Verification items for the finished model (mm, model axes). A direction names the side the tool comes from. Give positions to 0.01 mm unless a question says otherwise; leave off trailing zeros. Write each loop counter-clockwise with the first axis right and the second up, starting at its lowest first coordinate (ties: lowest second). Pieces come first, ordered by that corner, then holes.
Autodesk Inventor part; units mm, degrees
ref_plane "YZ Plane" through (0, 0, 0) normal (1, 0, 0) x (0, 1, 0)
ref_plane "XZ Plane" through (0, 0, 0) normal (0, 1, 0) x (-1, 0, 0)
ref_plane "XY Plane" through (0, 0, 0) normal (0, 0, 1) x (1, 0, 0)
sketch "Sketch1" plane through (0, 0, 0) normal (0, 1, 0) x (-1, 0, 0)
  line L0 (0, 18.5) -> (0, -18.5)
  line L1 (-4, 14.5) -> (-4, -14.5)
  line L2 (0, 0) -> (-19.6483, 0) construction
  line L3 (-4, 14.5) -> (0, 18.5)
  line L4 (0, -18.5) -> (-4, -14.5)
  point P0 (-4, 0)
  dimension "d6" = 37
  dimension "d7" = 29
  dimension "d8" = 4
extrude "Extrusion1" add sketch "Sketch1" along normal blind 18
sketch "Sketch2" plane through (4, 0, 14.5) normal (1, 0, 0) x (0, 0, -1)
  line L0 (-4, 0) -> (-4, 18)
  line L1 (33, 0) -> (33, 18)
  line L2 (-4, 6) -> (33, 6)
  line L3 (33, 6) -> (33, 1.9)
  line L4 (33, 1.9) -> (-4, 1.9)
  line L5 (-4, 1.9) -> (-4, 6)
  line L6 (0, 0) -> (29, 0)
  point P0 (14.5, 0)
  point P1 (-4, 1.9)
  dimension "d11" = 4.1
  dimension "d12" = 1.9
extrude "Extrusion2" cut sketch "Sketch2" against normal blind 2
properties part number "long PDMS Chamber top-bottom"
Item 1: Sectioned sample at A-A on x = 3.1. Record the cut outline in (y, z), then the cut area to 3 significant figures.
Answer key:
outline: (0, -15.4) - (1.9, -15.4) - (1.9, 15.4) - (0, 15.4) - close; (6, -15.4) - (18, -15.4) - (18, 15.4) - (6, 15.4) - close
area: 428 mm2
Item 2: Sectioned sample at C-C on y = 2.5. Record the cut outline in (x, z), then the cut area to 3 significant figures.
Answer key:
outline: (0, -18.5) - (2, -16.5) - (2, 16.5) - (0, 18.5) - close
area: 70.0 mm2
Item 3: Set-up check for faces 1 (the face through (0, 9, 0)), 2 (the face through (3, 6, 0)): record each of +Z, -Z, +X, -X, +Y, -Y from which the full face is reachable in a straight line by a thin tool's end or side.
Answer key:
face 1: +Z, -Z, -X, +Y, -Y
face 2: +Z, -Z, +X
Item 4: Scan lines: line 1 along Y through (x, z) = (2.5, 0); line 2 along X through (y, z) = (2.5, -5); line 3 along Z through (x, y) = (1.5, 7.25). Record each from-to range of solid material in increasing order.
Answer key:
line 1: y = 0 to 1.9, 6 to 18
line 2: x = 0 to 2
line 3: z = -17 to 17
Item 5: Release check for a two-part mould opening along Y. For faces 3 (the face through (4, 12, 0)), 4 (the face through (2, 18, 0)), 5 (the face through (3, 1.9, 0)), 6 (the face through (2, 0, 0)) record: released by +Y, released by -Y, zero draft, split by the parting line, or undercut.
Answer key:
face 3: zero draft
face 4: released by +Y
face 5: undercut
face 6: released by -Y
Item 6: Depth check by flat-ended pin: pin 1 (1 mm diameter, centred on x = 2, y = 7, fed in from -Z). Enter the tip coordinate at first touch or a pass-through.
Answer key:
pin 1: stops at z = -17
Item 7: Sectioned sample at B-B on z = -15.5. Record the cut outline in (x, y), then the cut area to 3 significant figures.
Answer key:
outline: (0, 0) - (3, 0) - (3, 1.9) - (2, 1.9) - (2, 6) - (3, 6) - (3, 18) - (0, 18) - close
area: 49.9 mm2
Item 8: Sectioned sample at D-D on x = 1.25. Record the cut outline in (y, z).
Answer key:
outline: (0, -17.25) - (18, -17.25) - (18, 17.25) - (0, 17.25) - close
